from build123d import *

# Parameters (mm, degrees)
SKETCH1_R                = 25.8953
BOSS_EXTRUDE2_DEPTH      = 4.7625
FILLET1_R                = 3.175
SKETCH2_W                = 14.732
SKETCH2_H                = 10.414
CUT_EXTRUDE2_DEPTH       = 12.7
CIRPATTERN1_COUNT        = 7
SKETCH4_R                = 1.143
CUT_EXTRUDE4_DEPTH       = 9.525
CIRPATTERN2_COUNT        = 7
SKETCH5_R                = 3.175
CUT_EXTRUDE5_DEPTH       = 37.89266219
SKETCH6_R                = 2.159
CUT_EXTRUDE7_DEPTH       = 37.89266219
SKETCH7_R                = 4.064
CUT_EXTRUDE8_DEPTH       = 2.54
BOSS_EXTRUDE4_REACH      = 44.38
FILLET2_R                = 0.127
CIRPATTERN5_COUNT        = 7
FILLET2_OF_CIRPATTERN5_R = 0.127


with BuildPart() as part:
    # Sketch1 → Boss-Extrude2 (new body)
    with BuildSketch(Plane.XY):
        Circle(SKETCH1_R)
    extrude(amount=-BOSS_EXTRUDE2_DEPTH)

    # Fillet1
    fillet1_edges = [part.edges().sort_by_distance(p)[0] for p in [
        (-25.8953, 0, -4.7625),
    ]]
    fillet(fillet1_edges, radius=FILLET1_R)

    # Sketch2 → Cut-Extrude2 (cut)
    with BuildSketch(Plane.XY):
        with Locations((0, 21.9583)):
            Rectangle(SKETCH2_W, SKETCH2_H)
    cut_extrude2 = extrude(amount=-CUT_EXTRUDE2_DEPTH, mode=Mode.SUBTRACT)

    # CirPattern1: Cut-Extrude2 ×7 about axis
    cirpattern1_axis = Axis((0, 0, 0), (0, 0, 1))
    for i in range(1, CIRPATTERN1_COUNT):
        add(cut_extrude2.rotate(cirpattern1_axis, i * 360 / CIRPATTERN1_COUNT), mode=Mode.SUBTRACT)

    # Sketch4 → Cut-Extrude4 (cut, symmetric)
    with BuildSketch(Plane(origin=(0, 0, 0), x_dir=(0, 0, -1), z_dir=(1, 0, 0))):
        with Locations((0, 22.5933)):
            Circle(SKETCH4_R)
    cut_extrude4 = extrude(amount=CUT_EXTRUDE4_DEPTH, both=True, mode=Mode.SUBTRACT)

    # CirPattern2: Cut-Extrude4 ×7 about axis
    cirpattern2_axis = Axis((0, 0, 0), (0, 0, 1))
    for i in range(1, CIRPATTERN2_COUNT):
        add(cut_extrude4.rotate(cirpattern2_axis, i * 360 / CIRPATTERN2_COUNT), mode=Mode.SUBTRACT)

    # Sketch5 → Cut-Extrude5 (cut, through all)
    with BuildSketch(Plane.XY):
        Circle(SKETCH5_R)
    extrude(amount=-CUT_EXTRUDE5_DEPTH, mode=Mode.SUBTRACT)

    # Sketch6 → Cut-Extrude7 (cut, through all)
    with BuildSketch(Plane(origin=(0, 0, -4.7625), x_dir=(-1, 0, 0), z_dir=(0, 0, -1))):
        with Locations((0, -11.1125)):
            Circle(SKETCH6_R)
        with Locations((-9.6237073, 5.55625)):
            Circle(SKETCH6_R)
        with Locations((9.6237073, 5.55625)):
            Circle(SKETCH6_R)
    extrude(amount=-CUT_EXTRUDE7_DEPTH, mode=Mode.SUBTRACT)

    # Sketch7 → Cut-Extrude8 (cut)
    with BuildSketch(Plane(origin=(0, 0, -4.7625), x_dir=(-1, 0, 0), z_dir=(0, 0, -1))):
        with Locations((9.6237073, 5.55625)):
            Circle(SKETCH7_R)
        with Locations((0, -11.1125)):
            Circle(SKETCH7_R)
        with Locations((-9.6237073, 5.55625)):
            Circle(SKETCH7_R)
    extrude(amount=-CUT_EXTRUDE8_DEPTH, mode=Mode.SUBTRACT)

    # Sketch10 → Boss-Extrude4 (add, up to next)
    with BuildSketch(Plane.ZY.offset(-7.366), mode=Mode.PRIVATE) as boss_extrude4_sk1:
        with BuildLine():
            Line((-4.7625, 16.7513), (0, 16.7513))
            Line((0, 16.7513), (0, 16.8783))
            ThreePointArc((0, 16.8783), (-2.7025038, 17.55765722), (-4.7625, 19.434214887))
            Line((-4.7625, 19.434214887), (-4.7625, 16.7513))
        make_face()
    boss_extrude4_tool1 = extrude(boss_extrude4_sk1.sketch, amount=BOSS_EXTRUDE4_REACH, mode=Mode.PRIVATE) - part.part
    boss_extrude4 = boss_extrude4_tool1.solids().sort_by_distance((7.366, 17.489807, -3.452063))[0]
    add(boss_extrude4)

    # Fillet2
    fillet2_edges = [part.edges().sort_by_distance(p)[0] for p in [
        (0, 19.434214887, -4.7625),
    ]]
    fillet(fillet2_edges, radius=FILLET2_R)

    # CirPattern5: Boss-Extrude4 ×7 about axis
    cirpattern5_axis = Axis((0, 0, 0), (0, 0, 1))
    for i in range(1, CIRPATTERN5_COUNT):
        add(boss_extrude4.rotate(cirpattern5_axis, i * 360 / CIRPATTERN5_COUNT))

    # Fillet2 of CirPattern5
    fillet2_of_cirpattern5_edges = [part.edges().sort_by_distance(p)[0] for p in [
        (-15.194281036, 12.117034789, -4.7625),
        (-18.946958545, -4.324519647, -4.7625),
        (-8.432189822, -17.509622585, -4.7625),
        (8.432189822, -17.509622585, -4.7625),
        (18.946958545, -4.324519647, -4.7625),
        (15.194281036, 12.117034789, -4.7625),
    ]]
    fillet(fillet2_of_cirpattern5_edges, radius=FILLET2_OF_CIRPATTERN5_R)


solid = part.part
Read the model definition and answer for the solid it produces. Units are mm, in the model's axes. A direction names the side the tool comes from. Round coordinates to 2 decimals unless told otherwise and drop trailing zeros. Use a Markdown table: item, result.
1) Flat-ended cylindrical pins translate along their axes: pin 1 (9 mm diameter, centred on x = 8.5, y = 5, fed in from -Z); pin 2 (5 mm diameter, centred on x = -9.62, y = 5.56, fed in from -Z); pin 3 (0.9 mm diameter, centred on y = 23, z = -0.5, fed in from -X); pin 4 (1 mm diameter, centred on y = -20, z = -3.5, fed in from -X). Find the tip coordinate at first contact, or state that the pin passes through.
Answers follow:
| item | result |
|---|---|
| pin 1 | stops at z = -4.76 |
| pin 2 | stops at z = -2.22 |
| pin 3 | stops at x = -12.73 |
| pin 4 | stops at x = -1.7 |
2) For a pull along X with two mould halves and no side action, classify faces 4 (the cylindrical face through (-13.5, 6.78, -3.51)), 5 (the flat face through (-11.67, 18.73, -2.35)), 6 (the cylindrical face through (20.2, -16.2, -0.8)) as pulls with the +X half, pulls with the -X half, needs draft (parallel to the pull), parting line crosses it, or undercut.
Answers follow:
| item | result |
|---|---|
| face 4 | undercut |
| face 5 | pulls with the -X half |
| face 6 | pulls with the +X half |
3) Straight lines are drawn through the part: line 1 along X through (y, z) = (21.5, -2.85); line 2 along Y through (x, z) = (0, -3.85) (1 decimal); line 3 along X through (y, z) = (5, -0.7). For each, find the intervals that lie inside material, in ascending order. Write a range as [from, to].
Answers follow:
| item | result |
|---|---|
| line 1 | x = [-13.96, -7.37], [7.37, 13.96] |
| line 2 | y = [-24.9, -15.2], [-7, -3.2], [3.2, 18.4] |
| line 3 | x = [-25.41, -18.08], [-17.66, -11.71], [-7.54, 7.54], [11.71, 17.66], [18.08, 25.41] |
4) The part is cut by section A-A (x = 0). Give the number of separate pieces and of enclosed holes in the cut face, plus the area to 3 significant figures.
Answers follow:
| item | result |
|---|---|
| separate pieces | 3 |
| enclosed holes | 0 |
| area | 145 mm2 |
5) A tool of negligible diameter and unlimited length cuts with its end or side. For faces 1 (the flat face through (-11.738, 21.544, -0.436)), 2 (the flat face through (7.366, 21, -2)), 3 (the flat face through (-15.66, -15.54, -2.35)), from which of +Z, -Z, +X, -X, +Y, -Y can it reach the whole face along a straight path? Write none if from no direction.
Answers follow:
| item | result |
|---|---|
| face 1 | +Z |
| face 2 | +Z, +Y |
| face 3 | +Z, -Y |
